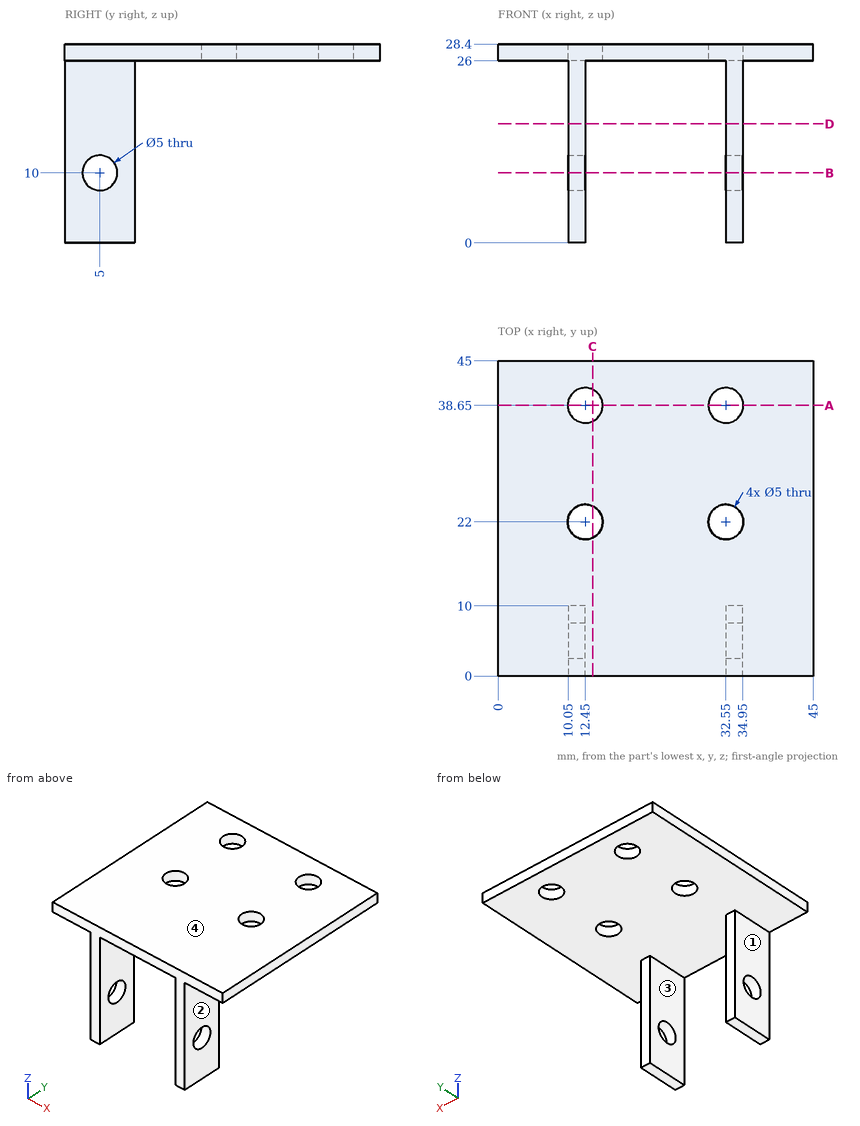
Design review of the part shown in the three views and the two pictorial views. Dimensions are in mm from the part's minimum x, y and z. A direction names the side the tool comes from. Round coordinates to 2 decimals unless told otherwise and drop trailing zeros. Loops run counter-clockwise (first coordinate to the right, second up) from the corner with the lowest first, then second, coordinate; pieces in that order, holes last. Notation, with made-up numbers: (82.25, -25) -> (120.25, -25) arc R20 ccw to (120.25, 12) -> close; hole circle Ø3 at (86.25, -35.75). An arc over 180 degrees is marked (long way). Use one line per item in the form item = value. Start each with the question number.
Q1. Machinability: for the marked faces 1, 2, 3 and 4, which of the approach directions +Z, -Z, +X, -X, +Y, -Y give a long, thin tool a straight path to every point of the face, cutting with its end or side? Answer none if there is none.
Q2. For pin 1 Ø3 at (y, z) = (39.5, 25) entering from -X; pin 2 Ø3 at (y, z) = (3.5, 16) entering from -X; pin 3 Ø5 at (x, z) = (36, 16) entering from +Y; pin 4 Ø8 at (x, y) = (12.45, 38.65) entering from -Z, all flat-tipped, find the tip position at first contact; note any pin that passes through.
Q3. We need section B-B on z = 10. Give the boundary of the cut face in (x, y).
Q4. Wall thickness on line 1 along Y through (x, z) = (12.45, 27.2); line 2 along Z through (x, y) = (33.75, 5); line 3 along Z through (x, y) = (8, 33.5): over which ranges is each line inside the solid? List them lowest first. Write a range as [from, to].
Q5. We need section C-C on x = 13.5. Give the boundary of the cut face in (y, z).
Q6. We need section A-A on y = 38.65. Give the boundary of the cut face in (x, z), then the cut area to 3 significant figures.
Q7. We need section D-D on z = 17. Give the boundary of the cut face in (x, y), then the cut area to 3 significant figures.
Calculated:
q1.face_1 = -Z, -X, +Y, -Y
q1.face_2 = -Z, +X, +Y, -Y
q1.face_3 = -Z, +Y, -Y
q1.face_4 = +Z, +X, -X, +Y, -Y
q2.pin_1 = 0
q2.pin_2 = 10.05
q2.pin_3 = 10
q2.pin_4 = 26
q3.outline = (10.05, 0) -> (12.45, 0) -> (12.45, 2.5) -> (10.05, 2.5) -> close; (10.05, 7.5) -> (12.45, 7.5) -> (12.45, 10) -> (10.05, 10) -> close; (32.55, 0) -> (34.95, 0) -> (34.95, 2.5) -> (32.55, 2.5) -> close; (32.55, 7.5) -> (34.95, 7.5) -> (34.95, 10) -> (32.55, 10) -> close
q4.line_1 = [0, 19.5], [24.5, 36.15], [41.15, 45]
q4.line_2 = [0, 7.5], [12.5, 28.4]
q4.line_3 = [26, 28.4]
q5.outline = (0, 26) -> (19.73, 26) -> (19.73, 28.4) -> (0, 28.4) -> close; (24.27, 26) -> (36.38, 26) -> (36.38, 28.4) -> (24.27, 28.4) -> close; (40.92, 26) -> (45, 26) -> (45, 28.4) -> (40.92, 28.4) -> close
q6.outline = (0, 26) -> (9.95, 26) -> (9.95, 28.4) -> (0, 28.4) -> close; (14.95, 26) -> (30.05, 26) -> (30.05, 28.4) -> (14.95, 28.4) -> close; (35.05, 26) -> (45, 26) -> (45, 28.4) -> (35.05, 28.4) -> close
q6.area = 84.0 mm²
q7.outline = (10.05, 0) -> (12.45, 0) -> (12.45, 10) -> (10.05, 10) -> close; (32.55, 0) -> (34.95, 0) -> (34.95, 10) -> (32.55, 10) -> close
q7.area = 48.0 mm²
